The figure shows three views and two pictorial views of one solid part (mm, origin at its lowest corner). Answer the questions. Round coordinates to 2 decimals unless told otherwise and drop trailing zeros. Write each loop counter-clockwise with the first axis right and the second up, starting at its lowest first coordinate (ties: lowest second). Pieces come first, ordered by that corner, then holes. Notation, with made-up numbers: (59.5, 12) -> (110.5, 12) arc R25 cw to (110.5, 40) -> close; hole circle Ø5 at (59, 22). An arc over 180 degrees is marked (long way). One line per item, written item: value.
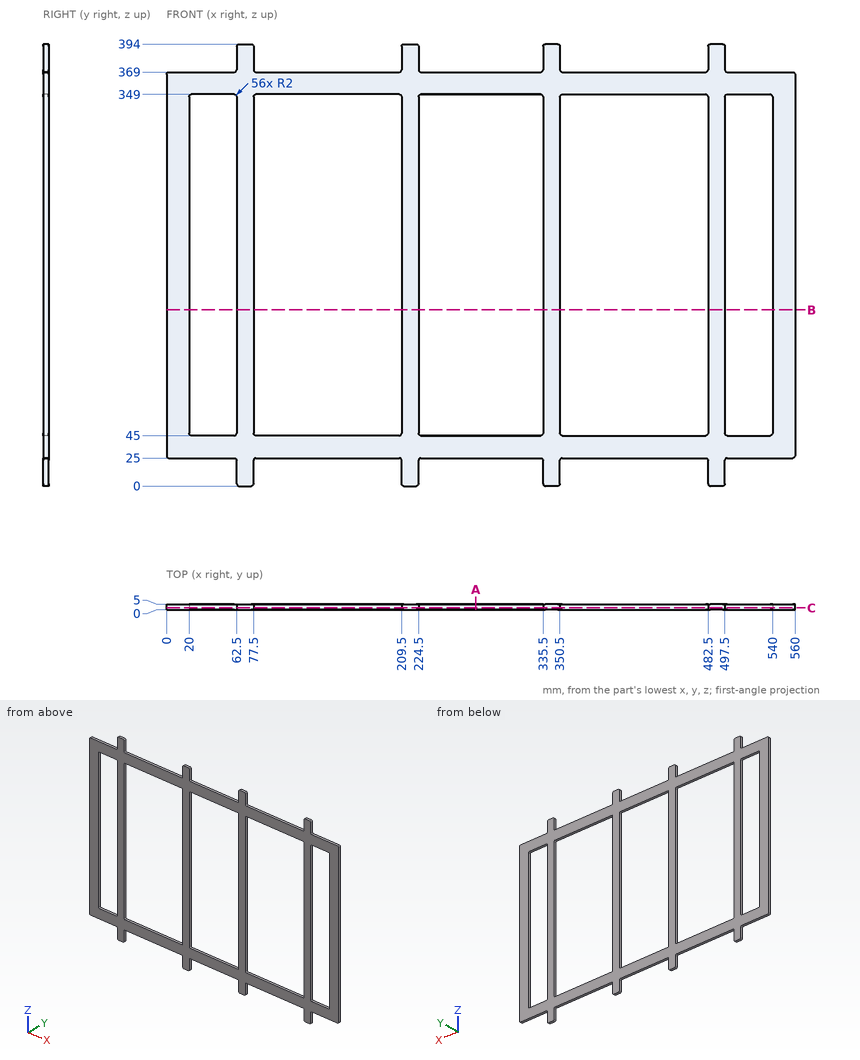
(1) Flat-ended cylindrical pins translate along their axes: pin 1 Ø1.5 at (y, z) = (2, 378) entering from -X; pin 2 Ø1.5 at (y, z) = (3.5, 378.5) entering from +X; pin 3 Ø1.5 at (x, y) = (328.5, 3) entering from -Z. Find the tip coordinate at first contact, or state that the pin passes through.
Reported:
pin 1: stops at x = 62.5
pin 2: stops at x = 497.5
pin 3: stops at z = 25
(2) Find section B-B on z = 157. Give the vertices of the cut face in (x, y).
Reported:
outline: (0, 0) -> (20, 0) -> (20, 5) -> (0, 5) -> close; (62.5, 0) -> (77.5, 0) -> (77.5, 5) -> (62.5, 5) -> close; (209.5, 0) -> (224.5, 0) -> (224.5, 5) -> (209.5, 5) -> close; (335.5, 0) -> (350.5, 0) -> (350.5, 5) -> (335.5, 5) -> close; (482.5, 0) -> (497.5, 0) -> (497.5, 5) -> (482.5, 5) -> close; (540, 0) -> (560, 0) -> (560, 5) -> (540, 5) -> close
(3) Find section C-C on y = 1.6. Give the number of separate pieces and of enclosed holes in the cut face, plus the area to 3 significant figures.
Reported:
separate pieces: 1
enclosed holes: 5
area: 55,800 mm2
(4) Find section A-A on x = 275.5. Give the vertices of the cut face in (y, z).
Reported:
outline: (0, 25) -> (5, 25) -> (5, 45) -> (0, 45) -> close; (0, 349) -> (5, 349) -> (5, 369) -> (0, 369) -> close
(5) Consider probe 1 along X at (y, z) = (3.8, 74); probe 2 along Z at (x, y) = (363, 0.55); probe 3 along Z at (x, y) = (223.5, 4.6). Determine where each line is inside the solid, lowest interval first.
Reported:
probe 1: x = 0 to 20, 62.5 to 77.5, 209.5 to 224.5, 335.5 to 350.5, 482.5 to 497.5, 540 to 560
probe 2: z = 25 to 45, 349 to 369
probe 3: z = 0.27 to 393.73
